Read the model definition and answer for the solid it produces. Units are mm, in the model's axes. Face numbers are marked on the shaded views. A direction names the side the tool comes from. Coordinates: 2 decimals unless noted, no trailing zeros. Write each loop counter-clockwise with the first axis right and the second up, starting at its lowest first coordinate (ties: lowest second). Pieces come first, ordered by that corner, then holes.
(1) Find the intervals of material crossed by probe 1 along Z at (x, y) = (121, 9); probe 2 along Z at (x, y) = (99.5, 67.5); probe 3 along Y at (x, z) = (67, -43.5), in increasing order.
(2) Section A-A on y = 22.5 is taken. Write down the section's boundary in (x, z).
(3) Which of the six approach directions +Z, -Z, +X, -X, +Y, -Y give full straight-line access (tool end or side, diameter ignored) to the marked faces 1 and 2?
(4) Given pin 1 (10 mm diameter, centred on x = 128, y = 38.5, fed in from -Z); pin 2 (4 mm diameter, centred on y = 42.5, z = -27, fed in from +X); pin 3 (24 mm diameter, centred on x = 95, y = 47.5, fed in from -Z), each flat-ended and moving along its own axis, determine where each tip first touches the part or whether it passes through.
(5) Section C-C on x = 50 is taken. Write down the section's boundary in (y, z), then the cut area to 3 significant figures.
(6) The mould has two halves that part along X. Classify the marked faces 3, 4 and 5: +X half, -X half, draft (parallel to the pull), parting line (faces both ways), or undercut.
(7) Section B-B on z = -75 is taken. Write down the section's boundary in (x, y).
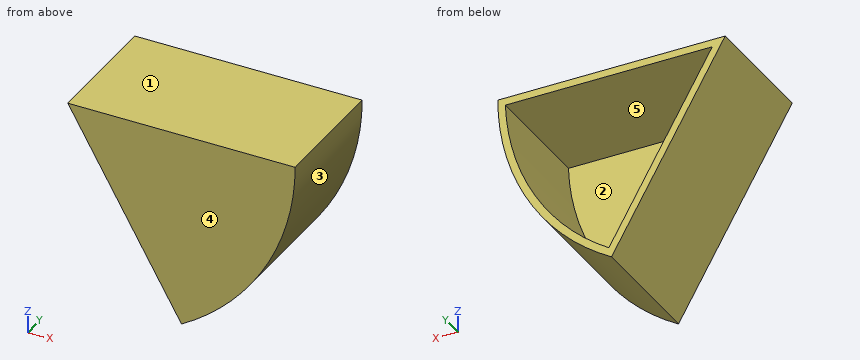
from build123d import *

# Parameters (mm, degrees)
EXTRUDE_1_DEPTH   = 5
EXTRUDE_1_2_DEPTH = 80


with BuildPart() as part:
    # 草图1 → Extrude 1 (new body)
    with BuildSketch(Plane(origin=(0, 0, 0), x_dir=(1, 0, 0), z_dir=(0, 1, 0))):
        with BuildLine():
            Line((0, 0), (153, 0))
            ThreePointArc((153, 0), (132.501886779, 76.5), (76.5, 132.501886779))
            Line((76.5, 132.501886779), (0, 0))
        make_face()
    extrude(amount=EXTRUDE_1_DEPTH)

    # 草图2 → Extrude 1 2 (add)
    with BuildSketch(Plane(origin=(0, 5, 0), x_dir=(1, 0, 0), z_dir=(0, 1, 0))):
        with BuildLine():
            Line((76.5, 132.501886779), (0, 0))
            Line((0, 0), (153, 0))
            ThreePointArc((153, 0), (132.501886779, 76.5), (76.5, 132.501886779))
        make_face()
        with BuildLine():
            Line((78.287885233, 125.59859484), (8.660254038, 5))
            Line((8.660254038, 5), (147.915516427, 5))
            ThreePointArc((147.915516427, 5), (128.17175976, 74), (78.287885233, 125.59859484))
        make_face(mode=Mode.SUBTRACT)
    extrude(amount=EXTRUDE_1_2_DEPTH)


solid = part.part
Response:
1. probe 1: z = -93.64 to -85.22, -5 to 0
1. probe 2: z = -116.23 to -109.56, -5 to 0
1. probe 3: y = 0 to 5
2. outline: (0, 0) - (76.5, -132.5) arc R153 ccw to (153, 0) - close; hole (8.66, -5) - (78.29, -125.6) arc R148 ccw to (147.92, -5) - close
3. face 1: +Z, +X, -X, +Y, -Y
3. face 2: +Y
4. pin 1: stops at z = -90.99
4. pin 2: stops at x = 150.94
4. pin 3: stops at z = -128.53
5. outline: (0, -86.6) - (85, -86.6) - (85, -76.6) - (5, -76.6) - (5, -5) - (85, -5) - (85, 0) - (0, 0) - close
5. area: 1,630 mm2
6. face 3: +X half
6. face 4: draft
6. face 5: undercut
7. outline: (43.3, 0) - (133.36, 0) - (133.36, 85) - (127.59, 85) - (127.59, 5) - (49.07, 5) - (49.07, 85) - (43.3, 85) - close
